```python
from build123d import *

# Parameters (mm, degrees)
EXTRUDE_1_DEPTH     = 8
SKETCH_2_R          = 2
CUT_EXTRUDE_1_DEPTH = 23.011360703
SKETCH_3_R          = 2
CUT_EXTRUDE_3_DEPTH = 8


with BuildPart() as part:
    # 草图1 → 凸台-拉伸1 (new body)
    with BuildSketch(Plane.XY):
        Polygon((0, 0), (14.5, 0), (14.5, 3), (3, 3), (3, 14.5), (0, 14.5), align=None)
    extrude(amount=EXTRUDE_1_DEPTH)

    # 草图2 → 切除-拉伸1 (cut, through all)
    with BuildSketch(Plane.XZ):
        with Locations(Location((8.5, 4, 0), (0, 0, 270))):
            Circle(SKETCH_2_R)
    extrude(amount=-CUT_EXTRUDE_1_DEPTH, mode=Mode.SUBTRACT)

    # 草图3 → 切除-拉伸3 (cut)
    with BuildSketch(Plane.ZY):
        with Locations((4, 8.5)):
            Circle(SKETCH_3_R)
    extrude(amount=-CUT_EXTRUDE_3_DEPTH, mode=Mode.SUBTRACT)


solid = part.part
```
Verification items for the finished model (mm, model axes). A direction names the side the tool comes from. Coordinates: 2 decimals unless noted, no trailing zeros. Loops run counter-clockwise (first coordinate to the right, second up) from the corner with the lowest first, then second, coordinate; pieces in that order, holes last. Notation, with made-up numbers: (-18, 69) - (-10, 69) arc R19 cw to (-10, 83) - close; hole circle Ø2 at (-15.5, 84.5). An arc over 180 degrees is marked (long way). Return JSON: item names as keys, results as strings.
1. Tool access check on faces 1 (the flat face through (2, 4, 8)), 2 (the flat face through (10, 3, 2)). Record the directions out of +Z, -Z, +X, -X, +Y, -Y that give a thin tool (end or side, any length) a straight path to the whole face; none if there is none.
Established:
{"face 1": "+Z, +X, -X, +Y, -Y", "face 2": "+Z, -Z, +X, +Y"}
2. Section check A-A, the plane x = 8.5. Record the boundary of the cut face in (y, z).
Established:
{"outline": "(0, 0) - (3, 0) - (3, 2) - (0, 2) - close; (0, 6) - (3, 6) - (3, 8) - (0, 8) - close"}
3. Mould release check, pull along Y, two halves, no side actions. Record for faces 3 (the flat face through (2, 14.5, 4)), 4 (the cylindrical face through (1.479, 10.483, 3.74)), 5 (the flat face through (14.5, 1, 4)): +Y half, -Y half, draft (parallel to the pull), parting line (faces both ways), or undercut.
Established:
{"face 3": "+Y half", "face 4": "undercut", "face 5": "draft"}
4. Section check C-C, the plane z = 4. Record the boundary of the cut face in (x, y).
Established:
{"outline": "(0, 0) - (6.5, 0) - (6.5, 3) - (3, 3) - (3, 6.5) - (0, 6.5) - close; (0, 10.5) - (3, 10.5) - (3, 14.5) - (0, 14.5) - close; (10.5, 0) - (14.5, 0) - (14.5, 3) - (10.5, 3) - close"}
5. Thickness scan on L1, parallel to Y at x = 2.2, z = 4; L2, parallel to Y at x = 12.75, z = 5. Record the ranges inside material, lowest first.
Established:
{"L1": "y = 0 to 6.5, 10.5 to 14.5", "L2": "y = 0 to 3"}
6. Section check D-D, the plane z = 7. Record the boundary of the cut face in (x, y).
Established:
{"outline": "(0, 0) - (14.5, 0) - (14.5, 3) - (3, 3) - (3, 14.5) - (0, 14.5) - close"}
7. Go/stop test with flat-tipped pins: pin 1 (2.5 mm diameter, centred on x = 11.5, z = 2.5, fed in from +Y); pin 2 (3 mm diameter, centred on x = 7.5, z = 2.5, fed in from -Y). Record where each tip stops, or that it passes through.
Established:
{"pin 1": "stops at y = 3", "pin 2": "stops at y = 0"}
